from build123d import *

# Parameters (mm, degrees)
SKETCH1_W                            = 80
SKETCH1_H                            = 73.57
BOSS_EXTRUDE1_DEPTH                  = 3
SKETCH2_W                            = 33
SKETCH2_H                            = 3
BOSS_EXTRUDE2_DEPTH                  = 25
F_4_0_4_DIAMETER_HOLE1_D             = 4
F_4_0_4_DIAMETER_HOLE1_DEPTH         = 8
F_4_0_4_DIAMETER_HOLE1_CSINK_D       = 4.05
F_4_0_4_DIAMETER_HOLE1_CSINK_ANGLE   = 90
F_4_0_4_DIAMETER_HOLE1_TIP           = 1.201721238
F_24_0_24_DIAMETER_HOLE1_D           = 24
F_24_0_24_DIAMETER_HOLE1_DEPTH       = 8
F_24_0_24_DIAMETER_HOLE1_CSINK_D     = 24.05
F_24_0_24_DIAMETER_HOLE1_CSINK_ANGLE = 90
F_24_0_24_DIAMETER_HOLE1_TIP         = 7.210327428
SKETCH11_W                           = 6
SKETCH11_H                           = 6.43
CUT_EXTRUDE2_DEPTH                   = 93.396624533
SKETCH12_W                           = 30
SKETCH12_H                           = 20
BOSS_EXTRUDE5_DEPTH                  = 290
CHAMFER3_SIZE                        = 15
CHAMFER3_SIZE2                       = 55.980762114
FILLET1_R                            = 10


with BuildPart() as part:
    # Sketch1 → Boss-Extrude1 (new, symmetric)
    with BuildSketch(Plane.XY):
        Rectangle(SKETCH1_W, SKETCH1_H)
    extrude(amount=BOSS_EXTRUDE1_DEPTH, both=True)

    # Sketch2 → Boss-Extrude2 (add)
    with BuildSketch(Plane.XY.offset(3)):
        with Locations((-23.5, -28.855)):
            Rectangle(SKETCH2_W, SKETCH2_H)
    extrude(amount=BOSS_EXTRUDE2_DEPTH)

    # Ø4.0 (4) Diameter Hole1
    with Locations(Plane(origin=(0, -27.355, 0), x_dir=(1, 0, 0), z_dir=(0, 1, 0))):
        with Locations((-33.5, -8), (-13.5, -8), (-13.5, -23), (-33.5, -23)):
            CounterSinkHole(F_4_0_4_DIAMETER_HOLE1_D / 2, F_4_0_4_DIAMETER_HOLE1_CSINK_D / 2, depth=F_4_0_4_DIAMETER_HOLE1_DEPTH, counter_sink_angle=F_4_0_4_DIAMETER_HOLE1_CSINK_ANGLE)
            with Locations((0, 0, -(F_4_0_4_DIAMETER_HOLE1_DEPTH + F_4_0_4_DIAMETER_HOLE1_TIP / 2))):  # 118° drill point
                Cone(0, F_4_0_4_DIAMETER_HOLE1_D / 2, F_4_0_4_DIAMETER_HOLE1_TIP, mode=Mode.SUBTRACT)

    # Ø24.0 (24) Diameter Hole1
    with Locations(Plane.XY.offset(3)):
        with Locations((15, -14.855)):
            CounterSinkHole(F_24_0_24_DIAMETER_HOLE1_D / 2, F_24_0_24_DIAMETER_HOLE1_CSINK_D / 2, depth=F_24_0_24_DIAMETER_HOLE1_DEPTH, counter_sink_angle=F_24_0_24_DIAMETER_HOLE1_CSINK_ANGLE)
            with Locations((0, 0, -(F_24_0_24_DIAMETER_HOLE1_DEPTH + F_24_0_24_DIAMETER_HOLE1_TIP / 2))):  # 118° drill point
                Cone(0, F_24_0_24_DIAMETER_HOLE1_D / 2, F_24_0_24_DIAMETER_HOLE1_TIP, mode=Mode.SUBTRACT)

    # Sketch11 → Cut-Extrude2 (cut, through all)
    with BuildSketch(Plane.ZY.offset(40)):
        with Locations((0, -33.57)):
            Rectangle(SKETCH11_W, SKETCH11_H)
    extrude(amount=-CUT_EXTRUDE2_DEPTH, mode=Mode.SUBTRACT)

    # Sketch12 → Boss-Extrude5 (add)
    with BuildSketch(Plane.XY.offset(3)):
        with Locations((15, 26.785)):
            Rectangle(SKETCH12_W, SKETCH12_H)
    extrude(amount=BOSS_EXTRUDE5_DEPTH)

    # Chamfer3
    chamfer3_edges = [part.edges().sort_by_distance(p)[0] for p in [
        (15, 16.785, 3),
    ]]
    chamfer3_side = [part.faces().sort_by_distance(p)[0] for p in [
        (-3.197697434, 2.561053146, 3),
    ]]
    chamfer(chamfer3_edges, length=CHAMFER3_SIZE, length2=CHAMFER3_SIZE2, reference=chamfer3_side[0])

    # Fillet1
    fillet1_edges = [part.edges().sort_by_distance(p)[0] for p in [
        (0, 19.285, 3),
        (30, 19.285, 3),
    ]]
    fillet(fillet1_edges, radius=FILLET1_R - 0.0001)  # a hair under: the kernel refuses the full size


solid = part.part
Design review of the part built by this model. Coordinates are the model's own, in mm. A direction names the side the tool comes from. Give positions to 0.01 mm unless a question says otherwise; leave off trailing zeros. Loops run counter-clockwise (first coordinate to the right, second up) from the corner with the lowest first, then second, coordinate; pieces in that order, holes last. Notation, with made-up numbers: M 42,-5.5 L 79,-5.5 A29 ccw 79,14.5 Z; hole C 25,89.5 d7. An arc over 180 degrees is marked long. Answer as a JSON object with one key per item and string values.
Item 1: We need section C-C (x = -3). State the section outline as (y, z) points (3 decimals).
Output values:
{"outline": "M -30.355,-3 L 36.785,-3 L 36.785,5.859 L 2.551,5.859 L 1.785,3 L -30.355,3 Z"}
Item 2: Machinability: for faces 5 (the face through (-3.01, 19.53, 5.85)), 6 (the face through (0, 24, 151)), 7 (the face through (15, 16.785, 174)), which of the approach directions +Z, -Z, +X, -X, +Y, -Y give a long, thin tool a straight path to every point of the face, cutting with its end or side? Answer none if there is none.
Output values:
{"face 5": "+Z, -X, +Y", "face 6": "+Z, -X, +Y, -Y", "face 7": "+Z, +X, -X, -Y"}
Item 3: For P1, Ø1.5, axis at x = -30, y = -29, coming from the +Z side; P2, Ø8, axis at x = 6, z = 81, coming from the -Y side (3 decimals); P3, Ø5, axis at x = -13.5, z = 23, coming from the +Y side (3 decimals); P4, Ø3, axis at x = -33.5, z = 8, coming from the -Y side, all flat-tipped, find the tip position at first contact; note any pin that passes through.
Output values:
{"P1": "stops at z = 28", "P2": "stops at y = 16.785", "P3": "stops at y = -27.355", "P4": "passes through"}
Item 4: Wall thickness on line 1 along X through (y, z) = (-28, 8); line 2 along Z through (x, y) = (-13.5, -28.9); line 3 along Z through (x, y) = (-13, -28): over which ranges is each line inside the solid? List them lowest first.
Output values:
{"line 1": "x = -40 to -35.5, -31.5 to -15.5, -11.5 to -7", "line 2": "z = -3 to 6, 10 to 21, 25 to 28", "line 3": "z = -3 to 6.06, 9.94 to 21.06, 24.94 to 28"}
Item 5: Mouldability with a two-part tool opening along X and no side actions: class faces 1 (the face through (8.549, -4.737, -0.054)), 2 (the face through (30, 24, 151)), 3 (the face through (-18, -30.355, 9)), 4 (the face through (-40, -2, 1)) as pulls with the +X half, pulls with the -X half, needs draft (parallel to the pull), parting line crosses it, or undercut.
Output values:
{"face 1": "undercut", "face 2": "pulls with the +X half", "face 3": "needs draft", "face 4": "pulls with the -X half"}
Item 6: We need section D-D (z = 50.5). State the section outline as (x, y) points (3 decimals), and give its area (3 significant figures).
Output values:
{"outline": "M 0,14.513 L 30,14.513 L 30,36.785 L 0,36.785 Z", "area": "668 mm2"}
Item 7: We need section B-B (z = 211). State the section outline as (x, y) points (3 decimals).
Output values:
{"outline": "M 0,16.785 L 30,16.785 L 30,36.785 L 0,36.785 Z"}
Item 8: We need section A-A (x = 15). State the section outline as (y, z) points (3 decimals), and give its area (3 significant figures).
Output values:
{"outline": "M -30.355,-3 L -26.855,-3 L -26.855,2.975 L -26.88,3 L -30.355,3 Z; M -2.855,-3 L 36.785,-3 L 36.785,293 L 16.785,293 L 16.785,58.981 L 1.785,3 L -2.83,3 L -2.855,2.975 Z", "area": "6,480 mm2"}
